The figure shows three views and two pictorial views of one solid part (mm, origin at its lowest corner). Answer the questions. Coordinates: 2 decimals unless noted, no trailing zeros. Write each loop counter-clockwise with the first axis right and the second up, starting at its lowest first coordinate (ties: lowest second). Pieces come first, ordered by that corner, then holes. Notation, with made-up numbers: M 88.5,76 L 122.5,76 A24 ccw 122.5,103 Z; hole C -4.5,-23.75 d1. An arc over 180 degrees is marked long. Write item = value, one per line. Start each with the question number.
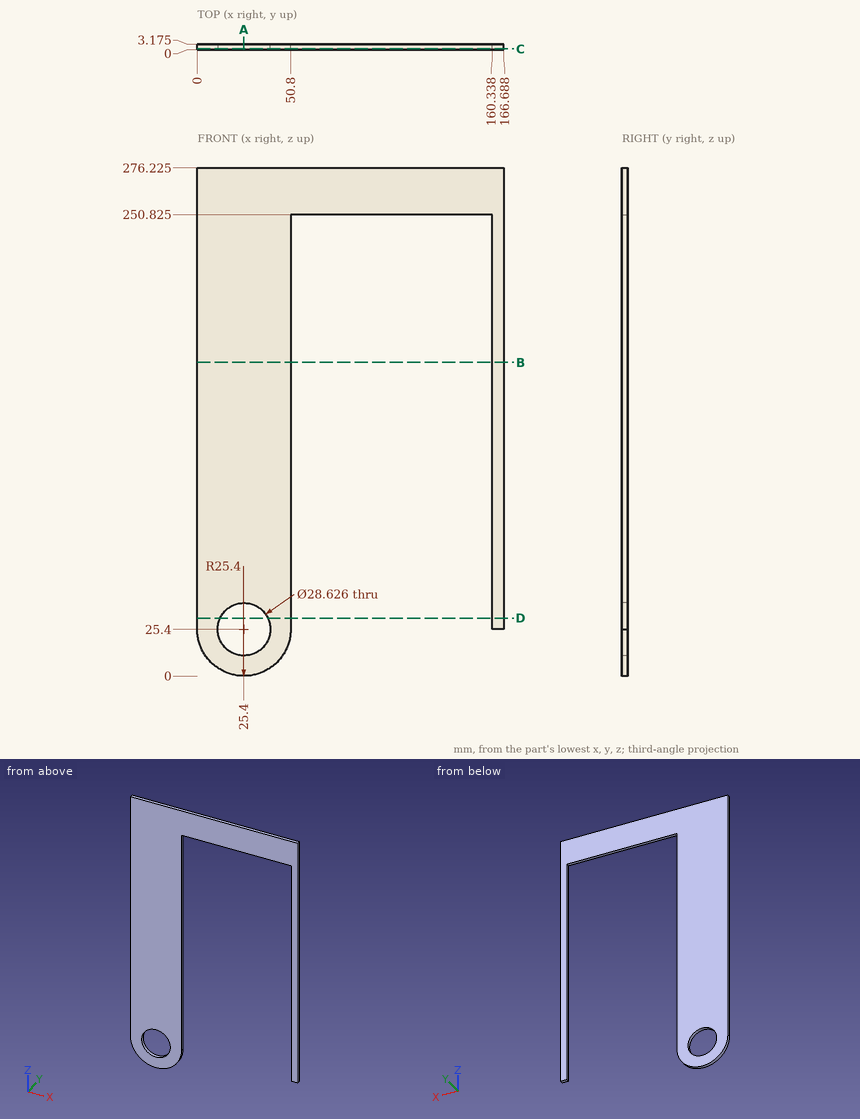
1. The part is cut by section A-A, the plane x = 25.4. Write down the section's boundary in (y, z) (1 decimal).
2. The part is cut by section C-C, the plane y = 0.5. Write down the section's boundary in (x, z) (1 decimal), and give its area (3 significant figures).
3. The part is cut by section B-B, the plane z = 170.5. Write down the section's boundary in (x, y) (1 decimal).
4. The part is cut by section D-D, the plane z = 31.5. Write down the section's boundary in (x, y) (1 decimal).
5. Straight lines are drawn through the part: L1, parallel to X at y = 1.7, z = 79.5; L2, parallel to Z at x = 25.4, y = 0.75 (1 decimal); L3, parallel to Z at x = 64.5, y = 0.65 (1 decimal). For each, find the intervals that lie inside material, in ascending order. Write a range as [from, to].
6. This flat-tipped pin is pushed along its axis until it touches: pin 1 (1 mm diameter, centred on x = 94, y = 2.5, fed in from -Z) (1 decimal). Where does it stop, or does it pass through?
Solution:
q1.outline = M 0,0 L 3.2,0 L 3.2,11.1 L 0,11.1 Z; M 0,39.7 L 3.2,39.7 L 3.2,276.2 L 0,276.2 Z
q2.outline = M 0,25.4 A25.4 ccw 50.8,25.4 L 50.8,250.8 L 160.3,250.8 L 160.3,25.4 L 166.7,25.4 L 166.7,276.2 L 0,276.2 Z; hole C 25.4,25.4 d28.6
q2.area = 17,500 mm^2
q3.outline = M 0,0 L 50.8,0 L 50.8,3.2 L 0,3.2 Z; M 160.3,0 L 166.7,0 L 166.7,3.2 L 160.3,3.2 Z
q4.outline = M 0,0 L 12.5,0 L 12.5,3.2 L 0,3.2 Z; M 38.3,0 L 50.8,0 L 50.8,3.2 L 38.3,3.2 Z; M 160.3,0 L 166.7,0 L 166.7,3.2 L 160.3,3.2 Z
q5.L1 = [0, 50.8], [160.34, 166.69]
q5.L2 = [0, 11.1], [39.7, 276.2]
q5.L3 = [250.8, 276.2]
q6.pin_1 = 250.8
